from build123d import *

# Parameters (mm, degrees)
SKETCH1_W           = 51
SKETCH1_H           = 77
BOSS_EXTRUDE1_DEPTH = 1.2
SKETCH2_R           = 1.77
CUT_EXTRUDE1_DEPTH  = 1.2
SKETCH3_W           = 13.21357214
SKETCH3_H           = 8.024996692
SKETCH3_W_2         = 15.358183325
SKETCH3_H_2         = 8.647625746
BOSS_EXTRUDE2_DEPTH = 15
SKETCH4_W           = 4.220041364
SKETCH4_H           = 15.634907348
SKETCH4_W_2         = 6.018747519
SKETCH4_H_2         = 16.603441432
BOSS_EXTRUDE3_DEPTH = 12


with BuildPart() as part:
    # Sketch1 → Boss-Extrude1 (new body)
    with BuildSketch(Plane(origin=(0, 0, 0), x_dir=(1, 0, 0), z_dir=(0, 1, 0))):
        with Locations((25.5, -38.5)):
            Rectangle(SKETCH1_W, SKETCH1_H)
    extrude(amount=BOSS_EXTRUDE1_DEPTH)

    # Sketch2 → Cut-Extrude1 (cut)
    with BuildSketch(Plane(origin=(0, 1.2, 0), x_dir=(1, 0, 0), z_dir=(0, 1, 0))):
        with Locations(Location((3.77, -3.77, 0), (0, 0, 270))):
            Circle(SKETCH2_R)
        with Locations(Location((46.77, -3.77, 0), (0, 0, 270))):
            Circle(SKETCH2_R)
        with Locations(Location((46.77, -73.77, 0), (0, 0, 270))):
            Circle(SKETCH2_R)
        with Locations(Location((3.77, -73.77, 0), (0, 0, 270))):
            Circle(SKETCH2_R)
    extrude(amount=-CUT_EXTRUDE1_DEPTH, mode=Mode.SUBTRACT)

    # Sketch3 → Boss-Extrude2 (add)
    with BuildSketch(Plane(origin=(0, 1.2, 0), x_dir=(1, 0, 0), z_dir=(0, 1, 0))):
        with Locations((26.088038551, -15.42813451)):
            Rectangle(SKETCH3_W, SKETCH3_H)
        with Locations((26.606896096, -27.846125081)):
            Rectangle(SKETCH3_W_2, SKETCH3_H_2)
    extrude(amount=BOSS_EXTRUDE2_DEPTH)

    # Sketch4 → Boss-Extrude3 (add)
    with BuildSketch(Plane(origin=(0, 1.2, 0), x_dir=(1, 0, 0), z_dir=(0, 1, 0))):
        with Locations((8.031795993, -21.170158005)):
            Rectangle(SKETCH4_W, SKETCH4_H)
        with Locations((41.861307912, -21.654425047)):
            Rectangle(SKETCH4_W_2, SKETCH4_H_2)
    extrude(amount=BOSS_EXTRUDE3_DEPTH)


solid = part.part
Geometry: final body of the model. Coordinates: model frame, mm. A direction names the side the tool comes from. Round coordinates to 2 decimals unless told otherwise and drop trailing zeros. Loops run counter-clockwise (first coordinate to the right, second up) from the corner with the lowest first, then second, coordinate; pieces in that order, holes last.
Q1. Pin query (flat end, axial travel): P1, Ø2, axis at y = 5.5, z = 19.5, coming from the -X side; P2, Ø3, axis at x = 23.5, z = 43, coming from the +Y side; P3, Ø1, axis at x = 33.5, y = 3, coming from the -Z side. Return the tip coordinate at first contact, or that it passes through.
Q2. Pull-direction query (Z, two-part tool) for faces 1 (the flat face through (26, 9, 11.416)), 2 (the flat face through (42, 7, 29.956)), 3 (the flat face through (34.286, 9, 28)), 4 (the flat face through (26, 9, 19.441)); classes: released by +Z, released by -Z, zero draft, split by the parting line, or undercut.
Q3. Section D-D on x = 27. Return loops of the section in (y, z).
Q4. Access query for faces 5 (the flat face through (5.922, 7, 21)), 6 (the flat face through (44.871, 7, 22)), 7 (the flat face through (10.142, 7, 21)). Directions: +Z, -Z, +X, -X, +Y, -Y. A direction counts if a zero-diameter tool reaches every point of the face in a straight line with its end or side. Return the directions, or none.
Q5. Material intervals for L1, parallel to X at y = 0.3, z = 73.77; L2, parallel to X at y = 12, z = 18; L3, parallel to X at y = 11.5, z = 23, sorted ascending.
Q6. Section B-B on x = 3.77. Return loops of the section in (y, z), plus the area to 3 significant figures.
Q7. Section A-A on y = 7.75. Return loops of the section in (x, z).
Q8. Section C-C on z = 73.77. Return loops of the section in (x, y).
Evaluation:
1. P1: stops at x = 5.92
1. P2: stops at y = 1.2
1. P3: stops at z = 23.52
2. face 1: released by -Z
2. face 2: released by +Z
2. face 3: zero draft
2. face 4: undercut
3. outline: (0, 0) - (1.2, 0) - (1.2, 11.42) - (16.2, 11.42) - (16.2, 19.44) - (1.2, 19.44) - (1.2, 23.52) - (16.2, 23.52) - (16.2, 32.17) - (1.2, 32.17) - (1.2, 77) - (0, 77) - close
4. face 5: +Z, -Z, -X, +Y
4. face 6: +Z, -Z, +X, +Y
4. face 7: +Z, -Z, +Y
5. L1: x = 0 to 2, 5.54 to 45, 48.54 to 51
5. L2: x = 5.92 to 10.14, 19.48 to 32.69, 38.85 to 44.87
5. L3: x = 5.92 to 10.14, 38.85 to 44.87
6. outline: (0, 0) - (1.2, 0) - (1.2, 2) - (0, 2) - close; (0, 5.54) - (1.2, 5.54) - (1.2, 72) - (0, 72) - close; (0, 75.54) - (1.2, 75.54) - (1.2, 77) - (0, 77) - close
6. area: 83.9 mm2
7. outline: (5.92, 13.35) - (10.14, 13.35) - (10.14, 28.99) - (5.92, 28.99) - close; (18.93, 23.52) - (34.29, 23.52) - (34.29, 32.17) - (18.93, 32.17) - close; (19.48, 11.42) - (32.69, 11.42) - (32.69, 19.44) - (19.48, 19.44) - close; (38.85, 13.35) - (44.87, 13.35) - (44.87, 29.96) - (38.85, 29.96) - close
8. outline: (0, 0) - (2, 0) - (2, 1.2) - (0, 1.2) - close; (5.54, 0) - (45, 0) - (45, 1.2) - (5.54, 1.2) - close; (48.54, 0) - (51, 0) - (51, 1.2) - (48.54, 1.2) - close
